Could you check a few things on this model? Use its own coordinates, in mm. Face numbers are marked on the shaded views. A direction names the side the tool comes from. Round coordinates to 2 decimals unless told otherwise and drop trailing zeros. Write each loop counter-clockwise with the first axis right and the second up, starting at its lowest first coordinate (ties: lowest second). Pieces come first, ordered by that corner, then holes. Notation, with made-up numbers: M 39,18.5 L 56,18.5 A28 ccw 56,36.5 Z; hole C 44,-9.5 d3. An arc over 180 degrees is marked long. One line per item, written item: value. Start each with the question number.
(1) I want a section at C-C on z = 29.5. Please give me the cut outline in (x, y), and give its area (3 significant figures).
(2) I want a section at A-A on z = 12. Count the separate pieces of the cut face and the enclosed holes in it, and give its area (3 significant figures).
(3) I want a section at B-B on x = -3. Please give me the cut outline in (y, z).
(4) I'm going to push flat-ended pins straight in: pin 1 Ø1.8 at (y, z) = (12.5, 29.5) entering from +X; pin 2 Ø0.6 at (x, y) = (29, 13) entering from +Z; pin 3 Ø6 at (y, z) = (-12, 24.5) entering from +X; pin 4 Ø0.8 at (x, y) = (16.5, -18.5) entering from +Z. Where does each tip first touch, or does it pass through?
(5) I want a section at D-D on x = 12. Please give me the cut outline in (y, z).
(6) Thinking about a two-plate mould opening in Y: for the marked faces 3, 4, 5 and 6, which applies, released by +Y, released by -Y, zero draft, split by the parting line, or undercut?
(7) If I drill on L1, parallel to Y at x = 44.8, z = 29.5; L2, parallel to Y at x = 29, z = 6.25; L3, parallel to X at y = 8, z = 2.5, over which ranges is the centre line in solid material (lowest first)?
(8) Which directions (+Z, -Z, +X, -X, +Y, -Y) give clear straight access to the entire face, cutting with the end or side of a thin tool? Please do the marked faces 1 and 2.
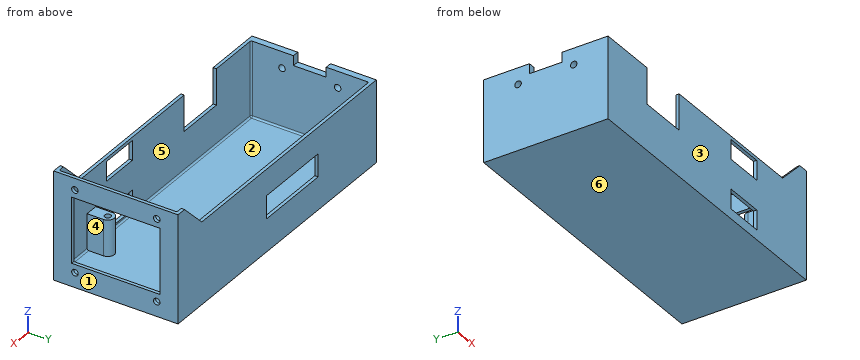
```python
from build123d import *

# Parameters (mm, degrees)
SKETCH_1_W          = 90
SKETCH_1_H          = 38
EXTRUDE_1_DEPTH     = 2
EXTRUDE_2_DEPTH     = 23
CUT_EXTRUDE_1_REACH = 65.984
SKETCH_3_W          = 12
SKETCH_3_H          = 6
SKETCH_3_W_2        = 15
SKETCH_3_H_2        = 11
CUT_EXTRUDE_2_REACH = 65.984
SKETCH_4_W          = 24
SKETCH_4_H          = 7
SKETCH_7_W          = 1
SKETCH_7_H          = 38
EXTRUDE_3_DEPTH     = 8
CUT_EXTRUDE_3_REACH = 99.724
SKETCH_6_W          = 20
SKETCH_6_H          = 27
CUT_EXTRUDE_4_REACH = 99.724
SKETCH_8_R          = 1
CHAMFER_1_SIZE      = 10
FILLET_1_R          = 0.5
SKETCH_10_R         = 0.95
EXTRUDE_4_DEPTH     = 11
SKETCH_11_R         = 1
EXTRUDE_5_DEPTH     = 2
FILLET_2_R          = 0.5


with BuildPart() as part:
    # 草图1 → 凸台-拉伸1 (new body)
    with BuildSketch(Plane.XY):
        Rectangle(SKETCH_1_W, SKETCH_1_H)
    extrude(amount=EXTRUDE_1_DEPTH)

    # 草图2 → 凸台-拉伸2 (add)
    with BuildSketch(Plane.XY.offset(2)):
        Polygon((44, 18), (-44, 18), (-45, 18), (-45, 19), (45, 19), (45, -19), (-45, -19), (-45, -18), (-44, -18), (44, -18), align=None)
    extrude(amount=EXTRUDE_2_DEPTH)

    # 草图3 → 切除-拉伸1 (cut, up to next)
    with BuildSketch(Plane.XZ.offset(19), mode=Mode.PRIVATE) as cut_extrude_1_sk1:
        with Locations((16, 6)):
            Rectangle(SKETCH_3_W, SKETCH_3_H)
    cut_extrude_1_tool1 = extrude(cut_extrude_1_sk1.sketch, amount=-CUT_EXTRUDE_1_REACH, mode=Mode.PRIVATE) & part.part
    # 草图3 → 切除-拉伸1 (cut, up to next)
    with BuildSketch(Plane.XZ.offset(19), mode=Mode.PRIVATE) as cut_extrude_1_sk2:
        with Locations((16, 21)):
            Rectangle(SKETCH_3_W, SKETCH_3_H)
    cut_extrude_1_tool2 = extrude(cut_extrude_1_sk2.sketch, amount=-CUT_EXTRUDE_1_REACH, mode=Mode.PRIVATE) & part.part
    # 草图3 → 切除-拉伸1 (cut, up to next)
    with BuildSketch(Plane.XZ.offset(19), mode=Mode.PRIVATE) as cut_extrude_1_sk3:
        with Locations((-21.5, 19.5)):
            Rectangle(SKETCH_3_W_2, SKETCH_3_H_2)
    cut_extrude_1_tool3 = extrude(cut_extrude_1_sk3.sketch, amount=-CUT_EXTRUDE_1_REACH, mode=Mode.PRIVATE) & part.part
    add(cut_extrude_1_tool1.solids().sort_by_distance((16, -19, 6))[0], mode=Mode.SUBTRACT)
    add(cut_extrude_1_tool2.solids().sort_by_distance((16, -19, 21))[0], mode=Mode.SUBTRACT)
    add(cut_extrude_1_tool3.solids().sort_by_distance((-21.5, -19, 19.5))[0], mode=Mode.SUBTRACT)

    # 草图4 → 切除-拉伸2 (cut, up to next)
    with BuildSketch(Plane(origin=(0, 19, 0), x_dir=(1, 0, 0), z_dir=(0, 1, 0)), mode=Mode.PRIVATE) as cut_extrude_2_sk1:
        with Locations((-8, -13.5)):
            Rectangle(SKETCH_4_W, SKETCH_4_H)
    cut_extrude_2_tool1 = extrude(cut_extrude_2_sk1.sketch, amount=-CUT_EXTRUDE_2_REACH, mode=Mode.PRIVATE) & part.part
    add(cut_extrude_2_tool1.solids().sort_by_distance((-8, 19, 13.5))[0], mode=Mode.SUBTRACT)

    # 草图7 → 凸台-拉伸3 (add)
    with BuildSketch(Plane.XY.offset(25)):
        with Locations((44.5, 0)):
            Rectangle(SKETCH_7_W, SKETCH_7_H)
    extrude(amount=EXTRUDE_3_DEPTH)

    # 草图6 → 切除-拉伸3 (cut, up to next)
    with BuildSketch(Plane(origin=(45, 0, 0), x_dir=(0, 0, -1), z_dir=(1, 0, 0)), mode=Mode.PRIVATE) as cut_extrude_3_sk1:
        with Locations((-17, 0)):
            Rectangle(SKETCH_6_W, SKETCH_6_H)
    cut_extrude_3_tool1 = extrude(cut_extrude_3_sk1.sketch, amount=-CUT_EXTRUDE_3_REACH, mode=Mode.PRIVATE) & part.part
    add(cut_extrude_3_tool1.solids().sort_by_distance((45, 0, 17))[0], mode=Mode.SUBTRACT)

    # 草图8 → 切除-拉伸4 (cut, up to next)
    with BuildSketch(Plane(origin=(45, 0, 0), x_dir=(0, 0, -1), z_dir=(1, 0, 0)), mode=Mode.PRIVATE) as cut_extrude_4_sk1:
        with Locations((-29.5, 12.5)):
            Circle(SKETCH_8_R)
    cut_extrude_4_tool1 = extrude(cut_extrude_4_sk1.sketch, amount=-CUT_EXTRUDE_4_REACH, mode=Mode.PRIVATE) & part.part
    # 草图8 → 切除-拉伸4 (cut, up to next)
    with BuildSketch(Plane(origin=(45, 0, 0), x_dir=(0, 0, -1), z_dir=(1, 0, 0)), mode=Mode.PRIVATE) as cut_extrude_4_sk2:
        with Locations((-29.5, -12.5)):
            Circle(SKETCH_8_R)
    cut_extrude_4_tool2 = extrude(cut_extrude_4_sk2.sketch, amount=-CUT_EXTRUDE_4_REACH, mode=Mode.PRIVATE) & part.part
    # 草图8 → 切除-拉伸4 (cut, up to next)
    with BuildSketch(Plane(origin=(45, 0, 0), x_dir=(0, 0, -1), z_dir=(1, 0, 0)), mode=Mode.PRIVATE) as cut_extrude_4_sk3:
        with Locations((-4.5, -12.5)):
            Circle(SKETCH_8_R)
    cut_extrude_4_tool3 = extrude(cut_extrude_4_sk3.sketch, amount=-CUT_EXTRUDE_4_REACH, mode=Mode.PRIVATE) & part.part
    # 草图8 → 切除-拉伸4 (cut, up to next)
    with BuildSketch(Plane(origin=(45, 0, 0), x_dir=(0, 0, -1), z_dir=(1, 0, 0)), mode=Mode.PRIVATE) as cut_extrude_4_sk4:
        with Locations((-4.5, 12.5)):
            Circle(SKETCH_8_R)
    cut_extrude_4_tool4 = extrude(cut_extrude_4_sk4.sketch, amount=-CUT_EXTRUDE_4_REACH, mode=Mode.PRIVATE) & part.part
    add(cut_extrude_4_tool1.solids().sort_by_distance((45, 12.5, 29.5))[0], mode=Mode.SUBTRACT)
    add(cut_extrude_4_tool2.solids().sort_by_distance((45, -12.5, 29.5))[0], mode=Mode.SUBTRACT)
    add(cut_extrude_4_tool3.solids().sort_by_distance((45, -12.5, 4.5))[0], mode=Mode.SUBTRACT)
    add(cut_extrude_4_tool4.solids().sort_by_distance((45, 12.5, 4.5))[0], mode=Mode.SUBTRACT)

    # 倒角1
    # the kernel refuses this chamfer: 10 mm, written as the material it adds along each edge
    with BuildSketch(Plane(origin=(44, 19, 25), x_dir=(-0.9996219169112968, 0, -0.027495876610586317), z_dir=(0, -1, 0))) as chamfer_1_piece_1_section:
        Polygon((CHAMFER_1_SIZE * 0.999621916911, -CHAMFER_1_SIZE * 0.0274958766106), (-CHAMFER_1_SIZE * 0.0274958766106, -CHAMFER_1_SIZE * 0.999621916911), (0, 0), align=None)
    chamfer_1_piece_1 = extrude(amount=1, mode=Mode.PRIVATE)
    chamfer_1_piece_1 = split(chamfer_1_piece_1, bisect_by=Plane(origin=(39.481481481, 18.5, 33), z_dir=(0, 0, -1)), keep=Keep.TOP, mode=Mode.PRIVATE)
    add(chamfer_1_piece_1)
    with BuildSketch(Plane(origin=(44, -18, 25), x_dir=(0.027495876610586317, 0, 0.9996219169112968), z_dir=(0, -1, 0))) as chamfer_1_piece_2_section:
        Polygon((CHAMFER_1_SIZE * 0.999621916911, CHAMFER_1_SIZE * 0.0274958766106), (-CHAMFER_1_SIZE * 0.0274958766106, CHAMFER_1_SIZE * 0.999621916911), (0, 0), align=None)
    chamfer_1_piece_2 = extrude(amount=1, mode=Mode.PRIVATE)
    chamfer_1_piece_2 = split(chamfer_1_piece_2, bisect_by=Plane(origin=(41.2, -18.5, 33), z_dir=(0, 0, -1)), keep=Keep.TOP, mode=Mode.PRIVATE)
    add(chamfer_1_piece_2)

    # 圆角1
    fillet_1_edges = [part.edges().sort_by_distance(p)[0] for p in [
        (-0.5, 18, 2),
        (44, 0, 2),
        (44, 18, 17.5),
        (-0.5, -18, 2),
        (44, -18, 17.5),
    ]]
    fillet(fillet_1_edges, radius=FILLET_1_R)

    # 草图10 → 凸台-拉伸4 (add)
    # profile 1 of 2: a face of its own
    with BuildSketch(Plane.XY.offset(2)):
        with BuildLine():
            Line((31, 13), (31, 18))
            Line((31, 18), (27, 18))
            Line((27, 18), (27, 13))
            ThreePointArc((27, 13), (29, 11), (31, 13))
        make_face()
        with Locations((29, 13)):
            Circle(SKETCH_10_R, mode=Mode.SUBTRACT)
    # profile 2 of 2: a face of its own
    with BuildSketch(Plane.XY.offset(2)):
        with BuildLine():
            Line((31, -13), (31, -18))
            Line((31, -18), (27, -18))
            Line((27, -18), (27, -13))
            ThreePointArc((27, -13), (29, -11), (31, -13))
        make_face()
        with Locations(Location((29, -13, 0), (0, 0, 180))):
            Circle(SKETCH_10_R, mode=Mode.SUBTRACT)
    extrude(amount=EXTRUDE_4_DEPTH)

    # 草图11 → 凸台-拉伸5 (add)
    with BuildSketch(Plane.ZY.offset(45)):
        Polygon((0, 19), (25, 19), (25, 5), (22, 5), (22, -5), (25, -5), (25, -19), (0, -19), align=None)
        with Locations(Location((20, 8.5, 0), (0, 0, 270))):
            Circle(SKETCH_11_R, mode=Mode.SUBTRACT)
        with Locations(Location((20, -8.5, 0), (0, 0, 270))):
            Circle(SKETCH_11_R, mode=Mode.SUBTRACT)
    extrude(amount=EXTRUDE_5_DEPTH)

    # 圆角2
    fillet_2_edges = [part.edges().sort_by_distance(p)[0] for p in [
        (-45, 18, 13.75),
        (-45, 0, 2),
        (-45, -17.853553391, 2.146446609),
        (-45, 17.853553391, 2.146446609),
        (-45, -18, 13.75),
    ]]
    fillet(fillet_2_edges, radius=FILLET_2_R)


solid = part.part
```
Found:
1. outline: M 38.5,-19 L 45,-19 L 45,-13.5 L 44,-13.5 L 44,-17.5 A0.5 cw 43.5,-18 L 38.5,-18 Z; M 38.5,18 L 43.5,18 A0.5 cw 44,17.5 L 44,13.5 L 45,13.5 L 45,19 L 38.5,19 Z; M 44,-11.5 L 45,-11.5 L 45,11.5 L 44,11.5 Z
1. area: 45.1 mm²
2. separate pieces: 2
2. enclosed holes: 2
2. area: 288 mm²
3. outline: M -19,0 L 19,0 L 19,10 L 18,10 L 18,2.5 A0.5 cw 17.5,2 L -17.5,2 A0.5 cw -18,2.5 L -18,25 L -19,25 Z; M 18,17 L 19,17 L 19,25 L 18,25 Z
4. pin 1: passes through
4. pin 2: stops at z = 2
4. pin 3: stops at x = 45
4. pin 4: stops at z = 25
5. outline: M -19,0 L 19,0 L 19,25 L 18,25 L 18,2.5 A0.5 cw 17.5,2 L -17.5,2 A0.5 cw -18,2.5 L -18,3 L -19,3 Z; M -19,9 L -18,9 L -18,18 L -19,18 Z; M -19,24 L -18,24 L -18,25 L -19,25 Z
6. face 3: released by -Y
6. face 4: undercut
6. face 5: undercut
6. face 6: zero draft
7. L1: y = -19 to -13.5, -11.5 to 11.5, 13.5 to 19
7. L2: y = -19 to -13.95, -12.05 to -11, 11 to 12.05, 13.95 to 19
7. L3: x = -47 to -45, 44 to 45
8. face 1: +Z, -Z, +X, +Y, -Y
8. face 2: +Z
